```python
from build123d import *

# Parameters (mm, degrees)
F0_R     = 3.175
F1_DEPTH = 1.190625
F2_DEPTH = 101.6


# Not quite as in the source:
# - a length typed as a fraction of an inch, garbled in the dataset ("3 / 203.2 mm" for 3/8 in), is restored


with BuildPart() as f1:
    # F0 (on Top) → F1 (new body)
    with BuildSketch(Plane.XY):
        with BuildLine():
            ThreePointArc((-3.7230175094, -0.5953125), (-3.7703125, 0), (-3.7230175094, 0.5953125))
            Line((-3.7230175094, 0.5953125), (-21.5030175094, 0.5953125))
            ThreePointArc((-21.5030175094, 0.5953125), (-21.0820680037, 0.4209495057), (-20.9077050094, 0))
            ThreePointArc((-20.9077050094, 0), (-21.0820680037, -0.4209495057), (-21.5030175094, -0.5953125))
            Line((-21.5030175094, -0.5953125), (-3.7230175094, -0.5953125))
        make_face()
        with BuildLine():
            ThreePointArc((-3.7230175094, -0.5953125), (0.2985941178, -3.7584701543), (3.7703125, 0))
            ThreePointArc((3.7703125, 0), (0.2985941178, 3.7584701543), (-3.7230175094, 0.5953125))
            ThreePointArc((-3.7230175094, 0.5953125), (-3.7703125, 0), (-3.7230175094, -0.5953125))
        make_face()
        Circle(F0_R, mode=Mode.SUBTRACT)
        with BuildLine():
            ThreePointArc((-20.9077050094, 0), (-21.0820680037, 0.4209495057), (-21.5030175094, 0.5953125))
            ThreePointArc((-21.5030175094, 0.5953125), (-22.0983300094, 0), (-21.5030175094, -0.5953125))
            ThreePointArc((-21.5030175094, -0.5953125), (-21.0820680037, -0.4209495057), (-20.9077050094, 0))
        make_face()
    extrude(amount=F1_DEPTH)

    # F0 (on Top) → F2 (join)
    with BuildSketch(Plane.XY):
        with BuildLine():
            ThreePointArc((-20.9077050094, 0), (-21.0820680037, 0.4209495057), (-21.5030175094, 0.5953125))
            ThreePointArc((-21.5030175094, 0.5953125), (-22.0983300094, 0), (-21.5030175094, -0.5953125))
            ThreePointArc((-21.5030175094, -0.5953125), (-21.0820680037, -0.4209495057), (-20.9077050094, 0))
        make_face()
    extrude(amount=-F2_DEPTH)


solid = f1.part
```
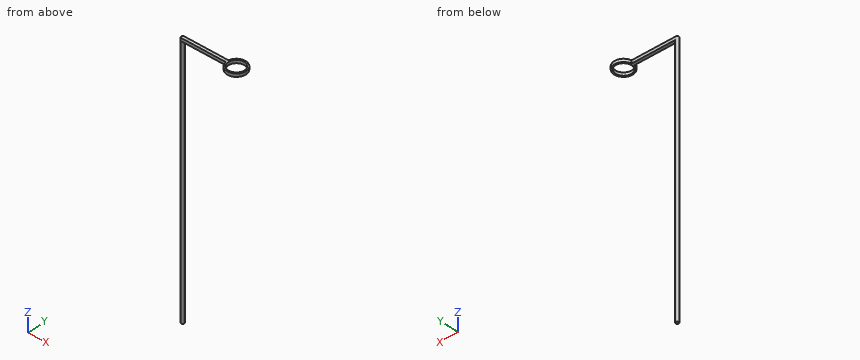
Check sheet for the modelled part. Datum: model origin and axes. Units: mm. Give positions to 0.01 mm unless a question says otherwise; leave off trailing zeros. Loops run counter-clockwise (first coordinate to the right, second up) from the corner with the lowest first, then second, coordinate; pieces in that order, holes last. Notation, with made-up numbers: M 21.25,18.5 L 31.25,18.5 A26 cw 31.25,42.5 Z; hole C 11.25,74 d10. An arc over 180 degrees is marked long. Answer in a Markdown table with one row per item.
1) Cross-section at C-C (z = -82.5). Enter the section's corners in (x, y).
Solutions:
| item | result |
|---|---|
| outline | C -21.5,0 d1.19 |
2) Thickness scan on line 1 (Y direction, x = 0, z = 0.75) (3 decimals); line 2 (Z direction, x = -6.25, y = -0.5); line 3 (X direction, y = -0.5, z = -11.5). Record the ranges inside material, lowest first.
Solutions:
| item | result |
|---|---|
| line 1 | y = -3.77 to -3.175, 3.175 to 3.77 |
| line 2 | z = 0 to 1.19 |
| line 3 | x = -21.83 to -21.18 |
3) Depth check by flat-ended pin: pin 1 (4 mm diameter, centred on x = 0, y = 0, fed in from -Z); pin 2 (1.3 mm diameter, centred on x = -11.5, z = 1, fed in from +Y). Enter the tip coordinate at first touch or a pass-through.
Solutions:
| item | result |
|---|---|
| pin 1 | passes through |
| pin 2 | stops at y = 0.6 |
4) Cross-section at A-A (x = 0). Enter the section's corners in (y, z) (3 decimals), plus the area to 3 significant figures.
Solutions:
| item | result |
|---|---|
| outline | M -3.77,0 L -3.175,0 L -3.175,1.191 L -3.77,1.191 Z; M 3.175,0 L 3.77,0 L 3.77,1.191 L 3.175,1.191 Z |
| area | 1.42 mm^2 |
5) Cross-section at B-B (x = -8.5). Enter the section's corners in (y, z), plus the area to 3 significant figures.
Solutions:
| item | result |
|---|---|
| outline | M -0.6,0 L 0.6,0 L 0.6,1.19 L -0.6,1.19 Z |
| area | 1.42 mm^2 |
